Read the model definition and answer for the solid it produces. Units are mm, in the model's axes. A direction names the side the tool comes from. Round coordinates to 2 decimals unless told otherwise and drop trailing zeros. Loops run counter-clockwise (first coordinate to the right, second up) from the corner with the lowest first, then second, coordinate; pieces in that order, holes last. Notation, with made-up numbers: M -40,68 L -3,68 A18 ccw -3,90 Z; hole C -25,27.25 d10. An arc over 180 degrees is marked long. Write each question's results on one line, items separated by ' | '.
```python
from build123d import *

# Parameters (mm, degrees)
BOSS_EXTRUDE1_DEPTH     = 6.8
SKETCH4_W               = 36
SKETCH4_H               = 8
BOSS_EXTRUDE2_DEPTH     = 2
SKETCH5_W               = 36
SKETCH5_H               = 4.1
BOSS_EXTRUDE3_DEPTH     = 6.8
CUT_EXTRUDE1_DEPTH      = 22.574058496
CUT_EXTRUDE1_DEPTH_BACK = 22.574058496
SKETCH6_R               = 1.65
FILLET3_R               = 0.35
FILLET4_R               = 1
CHAMFER1_SIZE           = 0.3


with BuildPart() as part:
    # Sketch1 → Boss-Extrude1 (new body)
    with BuildSketch(Plane(origin=(0, 0, 0), x_dir=(1, 0, 0), z_dir=(0, 1, 0))):
        Polygon((0, 0), (-18, 0), (-18, -2), (-16.8, -2), (-16.8, -3.15), (-16, -3.15), (-16, -2), (-14.8, -2), (-14.8, -3.15), (-14, -3.15), (-14, -2), (-12.8, -2), (-12.8, -3.15), (-12, -3.15), (-12, -2), (-10.8, -2), (-10.8, -3.15), (-10, -3.15), (-10, -2), (-8.8, -2), (-8.8, -3.15), (-8, -3.15), (-8, -2), (-6.8, -2), (-6.8, -3.15), (-6, -3.15), (-6, -2), (-4.8, -2), (-4.8, -3.15), (-4, -3.15), (-4, -2), (-2.8, -2), (-2.8, -3.15), (-2, -3.15), (-2, -2), (-0.8, -2), (-0.8, -3.15), (0, -3.15), (0, -2), (1.2, -2), (1.2, -3.15), (2, -3.15), (2, -2), (3.2, -2), (3.2, -3.15), (4, -3.15), (4, -2), (5.2, -2), (5.2, -3.15), (6, -3.15), (6, -2), (7.2, -2), (7.2, -3.15), (8, -3.15), (8, -2), (9.2, -2), (9.2, -3.15), (10, -3.15), (10, -2), (11.2, -2), (11.2, -3.15), (12, -3.15), (12, -2), (13.2, -2), (13.2, -3.15), (14, -3.15), (14, -2), (15.2, -2), (15.2, -3.15), (16, -3.15), (16, -2), (17.2, -2), (17.2, -3.15), (18, -3.15), (18, -2), (18, 0), align=None)
    extrude(amount=BOSS_EXTRUDE1_DEPTH)

    # Sketch4 → Boss-Extrude2 (add)
    with BuildSketch(Plane(origin=(0, 6.8, 0), x_dir=(1, 0, 0), z_dir=(0, 1, 0))):
        with Locations((0, -4)):
            Rectangle(SKETCH4_W, SKETCH4_H)
    extrude(amount=BOSS_EXTRUDE2_DEPTH)

    # Sketch5 → Boss-Extrude3 (add)
    with BuildSketch(Plane.XZ.offset(-6.8)):
        with Locations((0, 5.95)):
            Rectangle(SKETCH5_W, SKETCH5_H)
    extrude(amount=BOSS_EXTRUDE3_DEPTH)

    # Sketch6 → Cut-Extrude1 (cut, two sides: drawn at the far end of the back side and taken through both)
    with BuildSketch(Plane(origin=(0, 8.8, 0), x_dir=(1, 0, 0), z_dir=(0, 1, 0)).offset(-CUT_EXTRUDE1_DEPTH_BACK)):
        with Locations((-10, -6.65)):
            Circle(SKETCH6_R)
        with Locations((10, -6.65)):
            Circle(SKETCH6_R)
    extrude(amount=CUT_EXTRUDE1_DEPTH + CUT_EXTRUDE1_DEPTH_BACK, mode=Mode.SUBTRACT)

    # Fillet3
    fillet3_edges = [part.edges().sort_by_distance(p)[0] for p in [
        (9.051316702, 4.4, 8),
        (10.948683298, 4.4, 8),
        (-10.948683298, 4.4, 8),
        (-9.051316702, 4.4, 8),
    ]]
    fillet(fillet3_edges, radius=FILLET3_R)

    # Fillet4
    fillet4_edges = [part.edges().sort_by_distance(p)[0] for p in [
        (18, 4.4, 0),
        (-18, 4.4, 0),
        (-18, 4.4, 8),
        (18, 4.4, 8),
    ]]
    fillet(fillet4_edges, radius=FILLET4_R)

    # Chamfer1
    chamfer1_edges = [part.edges().sort_by_distance(p)[0] for p in [
        (14.366025404, 8.8, 8),
        (10, 8.8, 5),
        (-10, 8.8, 5),
        (0, 8.8, 8),
        (-11.428941916, 8.8, 7.825),
        (-8.571058084, 8.8, 7.825),
        (8.571058084, 8.8, 7.825),
        (11.428941916, 8.8, 7.825),
        (-14.366025404, 8.8, 8),
        (-18, 8.8, 4),
        (18, 8.8, 4),
        (0, 8.8, 0),
        (-17.707106781, 8.8, 0.292893219),
        (17.707106781, 8.8, 0.292893219),
        (17.707106781, 8.8, 7.707106781),
        (-17.707106781, 8.8, 7.707106781),
    ]]
    chamfer(chamfer1_edges, length=CHAMFER1_SIZE)


solid = part.part
```
1. Which of the six approach directions +Z, -Z, +X, -X, +Y, -Y give full straight-line access (tool end or side, diameter ignored) to faces 1 (the face through (11.2, 3.4, 2.6)), 2 (the face through (-16.4, 3.4, 3.15)), 3 (the face through (0, 4, 0))?
Completed:
face 1: -Y | face 2: +X, -X, -Y | face 3: -Z, +X, -X, +Y, -Y
2. Given P1, Ø0.6, axis at y = 4.5, z = 3, coming from the -X side; P2, Ø0.6, axis at x = 10.5, y = 4, coming from the +Z side, each flat-ended and moving along its own axis, determine where each tip first touches the part or whether it passes through.
Completed:
P1: stops at x = -16.8 | P2: stops at z = 5.21
3. Find section B-B, the plane z = 3.5. Give the vertices of the cut face in (x, y), then the cut area to 3 significant figures.
Completed:
outline: M -18,6.8 L 18,6.8 L 18,8.5 L 17.7,8.8 L -17.7,8.8 L -18,8.5 Z | area: 71.9 mm2
4. Find the intervals of material crossed by L1, parallel to X at y = 3.5, z = 6.65; L2, parallel to Z at x = 5, y = 3.25; L3, parallel to Z at x = 5.5, y = 5.5, in increasing order.
Completed:
L1: x = -18 to -11.65, -8.35 to 8.35, 11.65 to 18 | L2: z = 0 to 2, 3.9 to 8 | L3: z = 0 to 3.15, 3.9 to 8
5. Find section A-A, the plane z = 6.65. Give the vertices of the cut face in (x, y), then the cut area to 3 significant figures.
Completed:
outline: M -18,0 L -11.65,0 L -11.65,8.5 L -11.95,8.8 L -17.7,8.8 L -18,8.5 Z; M -8.35,0 L 8.35,0 L 8.35,8.5 L 8.05,8.8 L -8.05,8.8 L -8.35,8.5 Z; M 11.65,0 L 18,0 L 18,8.5 L 17.7,8.8 L 11.95,8.8 L 11.65,8.5 Z | area: 258 mm2
